CAD build for the part. Positions are in the model's coordinates, mm. Face numbers are marked on the shaded views. A direction names the side the tool comes from. Give positions to 0.01 mm unless a question says otherwise; leave off trailing zeros. Loops run counter-clockwise (first coordinate to the right, second up) from the corner with the lowest first, then second, coordinate; pieces in that order, holes last. Notation, with made-up numbers: M 30,45 L 46,45 A24 ccw 46,84 Z; hole C 81,11 d5. An arc over 180 degrees is marked long. One line per question, with ' | ' between items.
```python
from build123d import *

# Parameters (mm, degrees)
SKETCH086_R           = 2.5
PAD028_DEPTH          = 4
PAD029_DEPTH          = 14
SKETCH088_R           = 2.5
POCKET028_DEPTH       = 4.5
POLARPATTERN014_COUNT = 4
SKETCH089_R           = 5
SKETCH089_R_2         = 2.5
PAD030_DEPTH          = 4
FILLET_R              = 3


with BuildPart() as part:
    # Sketch086 → Pad028 (new body)
    with BuildSketch(Plane.XY):
        with BuildLine():
            Line((36.4, 15.2), (6.4, -24.8))
            ThreePointArc((-6.4, -24.8), (0, -28), (6.4, -24.8))
            Line((-6.4, -24.8), (-36.4, 15.2))
            ThreePointArc((-25.905574, 26.872821), (-35.949169, 25.348588), (-36.4, 15.2))
            Line((-25.905574, 26.872821), (-20.472131, 23.635893))
            ThreePointArc((-20.472131, 23.635893), (0, 18), (20.472131, 23.635893))
            Line((25.905574, 26.872821), (20.472131, 23.635893))
            ThreePointArc((36.4, 15.2), (35.949169, 25.348588), (25.905574, 26.872821))
        make_face()
        with Locations((30, 20)):
            Circle(SKETCH086_R, mode=Mode.SUBTRACT)
        with Locations((-30, 20)):
            Circle(SKETCH086_R, mode=Mode.SUBTRACT)
        with Locations((0, -20)):
            Circle(SKETCH086_R, mode=Mode.SUBTRACT)
        with BuildLine():
            Line((-9, -10), (9, -10))
            ThreePointArc((9, -10), (9.707107, -9.707107), (10, -9))
            Line((10, -9), (10, 9))
            ThreePointArc((10, 9), (9.707107, 9.707107), (9, 10))
            Line((9, 10), (-9, 10))
            ThreePointArc((-9, 10), (-9.707107, 9.707107), (-10, 9))
            Line((-10, 9), (-10, -9))
            ThreePointArc((-10, -9), (-9.707107, -9.707107), (-9, -10))
        make_face(mode=Mode.SUBTRACT)
    extrude(amount=PAD028_DEPTH)

    # Sketch087 (on Face21 of Pad028) → Pad029 (join)
    with BuildSketch(Plane.XY.offset(4)):
        with BuildLine():
            Line((-9, 13), (9, 13))
            ThreePointArc((13, 9), (11.828427, 11.828427), (9, 13))
            Line((13, 9), (13, -9))
            ThreePointArc((9, -13), (11.828427, -11.828427), (13, -9))
            Line((9, -13), (-9, -13))
            ThreePointArc((-13, -9), (-11.828427, -11.828427), (-9, -13))
            Line((-13, -9), (-13, 9))
            ThreePointArc((-9, 13), (-11.828427, 11.828427), (-13, 9))
        make_face()
        with BuildLine():
            Line((-9, -10), (9, -10))
            ThreePointArc((9, -10), (9.707107, -9.707107), (10, -9))
            Line((10, -9), (10, 9))
            ThreePointArc((10, 9), (9.707107, 9.707107), (9, 10))
            Line((9, 10), (-9, 10))
            ThreePointArc((-9, 10), (-9.707107, 9.707107), (-10, 9))
            Line((-10, 9), (-10, -9))
            ThreePointArc((-10, -9), (-9.707107, -9.707107), (-9, -10))
        make_face(mode=Mode.SUBTRACT)
    extrude(amount=PAD029_DEPTH)

    # Sketch088 → Pocket028 (cut, symmetric)
    with BuildSketch(Plane(origin=(0, 13, 0), x_dir=(-1, 0, 0), z_dir=(0, 1, 0))):
        with Locations((0, 10.5)):
            Circle(SKETCH088_R)
    pocket028 = extrude(amount=POCKET028_DEPTH, both=True, mode=Mode.SUBTRACT)

    # PolarPattern014: Pocket028 ×4 about axis
    polarpattern014_axis = Axis((0, 0, 0), (0, 0, 1))
    for i in range(1, POLARPATTERN014_COUNT):
        add(pocket028.rotate(polarpattern014_axis, i * 360 / POLARPATTERN014_COUNT), mode=Mode.SUBTRACT)

    # Sketch089 (on Face1 of PolarPattern014) → Pad030 (join)
    with BuildSketch(Plane.XY.offset(4)):
        with Locations((30, 20)):
            Circle(SKETCH089_R)
        with Locations((30, 20)):
            Circle(SKETCH089_R_2, mode=Mode.SUBTRACT)
        with Locations((-30, 20)):
            Circle(SKETCH089_R)
        with Locations((-30, 20)):
            Circle(SKETCH089_R_2, mode=Mode.SUBTRACT)
        with Locations((0, -20)):
            Circle(SKETCH089_R)
        with Locations((0, -20)):
            Circle(SKETCH089_R_2, mode=Mode.SUBTRACT)
    extrude(amount=PAD030_DEPTH)

    # Fillet
    fillet_edges = [part.edges().sort_by_distance(p)[0] for p in [
        (-11.828427, 11.828427, 4),
    ]]
    fillet(fillet_edges, radius=FILLET_R)


solid = part.part
```
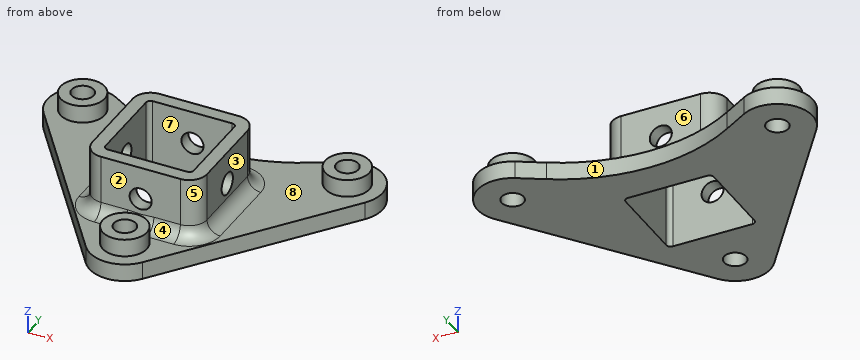
Item 1: 3-axis set-ups, long thin cutter, end or side, ignore diameter. For the marked faces 4, 5, 6, 7 and 8: which of +Z, -Z, +X, -X, +Y, -Y reach the whole face in a straight line?
Conclusion:
face 4: +Z, +X | face 5: +Z, +X, -Y | face 6: +Z, +X, -X, +Y | face 7: +Z, -Z | face 8: +Z
Item 2: Saw through at A-A on y = -8. Give the cut face in (x, z), and give its area (3 significant figures).
Conclusion:
outline: M -19,0 L -10,0 L -10,18 L -13,18 L -13,7 A3 cw -16,4 L -19,4 Z; M 10,0 L 19,0 L 19,4 L 16,4 A3 cw 13,7 L 13,18 L 10,18 Z | area: 160 mm²
Item 3: Mould opens along X. For the marked faces 1, 2 and 3 say: pulls with the +X half, pulls with the -X half, needs draft (parallel to the pull), parting line crosses it, or undercut.
Conclusion:
face 1: undercut | face 2: needs draft | face 3: pulls with the +X half
Item 4: Saw through at B-B on z = 12. State how many separate pieces and enclosed holes the cut face has, and give its area (3 significant figures).
Conclusion:
separate pieces: 4 | enclosed holes: 0 | area: 215 mm²
Item 5: Drill centre lines: line 1 along Z through (x, y) = (0, 11); line 2 along Y through (x, z) = (-0.5, 15.5); line 3 along Y through (x, z) = (30, 5.75). Where is each one in solid material? Low to high. Write a range as [from, to].
Conclusion:
line 1: [0, 8], [13, 18] | line 2: [-13, -10], [10, 13] | line 3: [15, 17.5], [22.5, 25]
Item 6: Saw through at C-C on y = 20. Give the cut face in (x, z), and give its area (3 significant figures).
Conclusion:
outline: M -38,0 L -32.5,0 L -32.5,8 L -35,8 L -35,4 L -38,4 Z; M -27.5,0 L -12.49,0 L -12.49,4 L -25,4 L -25,8 L -27.5,8 Z; M 12.49,0 L 27.5,0 L 27.5,8 L 25,8 L 25,4 L 12.49,4 Z; M 32.5,0 L 38,0 L 38,4 L 35,4 L 35,8 L 32.5,8 Z | area: 204 mm²
Item 7: Saw through at D-D on x = -30. Give the cut face in (y, z).
Conclusion:
outline: M 6.67,0 L 17.5,0 L 17.5,8 L 15,8 L 15,4 L 6.67,4 Z; M 22.5,0 L 28,0 L 28,4 L 25,4 L 25,8 L 22.5,8 Z
Item 8: Drop flat-ended pins along their axis: P1, Ø1, axis at y = 8.5, z = 14.5, coming from the -X side; P2, Ø6, axis at y = -10.5, z = 6.5, coming from the +X side; P3, Ø3, axis at x = -2, y = -22, coming from the +Z side; P4, Ø4.5, axis at x = 30, y = 20, coming from the +Z side. Give the stop position or say it passes through.
Conclusion:
P1: x = -13 | P2: x = 18.37 | P3: z = 8 | P4: through
